The model under review builds one solid part; all positions refer to its coordinate system, in mm. Face numbers are marked on the shaded views. A direction names the side the tool comes from. Coordinates: 2 decimals unless noted, no trailing zeros. Loops run counter-clockwise (first coordinate to the right, second up) from the corner with the lowest first, then second, coordinate; pieces in that order, holes last. Notation, with made-up numbers: M -21.5,35.5 L 21.5,35.5 A27 cw 21.5,64.5 Z; hole C 82,36 d11. An arc over 180 degrees is marked long. Return JSON: item names as keys, results as strings.
```python
from build123d import *

# Parameters (mm, degrees)
F0_R     = 4
F1_DEPTH = 6
F3_SIZE  = 0.5
F4_R     = 1
F2_R     = 3
F5_DEPTH = 25
F6_SIZE  = 1.5


with BuildPart() as f1:
    # F0 (on Front) → F1 (new body)
    with BuildSketch(Plane.XZ):
        Polygon((0, 7.5055534995), (-6.5, 3.7527767497), (-6.5, -3.7527767497), (0, -7.5055534995), (6.5, -3.7527767497), (6.5, 3.7527767497), align=None)
        Circle(F0_R, mode=Mode.SUBTRACT)
        Circle(F0_R)
    extrude(amount=-F1_DEPTH)

    # F3
    f3_edges = [f1.edges().sort_by_distance(p)[0] for p in [
        (6.5, 0, 0),
        (-3.25, 0, 5.629165),
        (-6.5, 0, 0),
        (-3.25, 0, -5.629165),
        (3.25, 0, -5.629165),
        (-3.25, 6, 5.629165),
        (-6.5, 6, 0),
        (-3.25, 6, -5.629165),
        (3.25, 6, -5.629165),
        (6.5, 6, 0),
        (3.25, 6, 5.629165),
    ]]
    chamfer(f3_edges, length=F3_SIZE)

    # F4
    f4_edges = [f1.edges().sort_by_distance(p)[0] for p in [
        (0, 3, 7.505553),
        (-6.5, 3, 3.752777),
        (6.5, 3, 3.752777),
        (-6.5, 3, -3.752777),
        (0, 3, -7.505553),
        (6.5, 3, -3.752777),
    ]]
    fillet(f4_edges, radius=F4_R)

    # F2 (on face) → F5 (join)
    with BuildSketch(Plane.XZ):
        Circle(F2_R)
    extrude(amount=F5_DEPTH)

    # F6
    f6_edges = [f1.edges().sort_by_distance(p)[0] for p in [
        (-3, -25, 0),
    ]]
    chamfer(f6_edges, length=F6_SIZE)


solid = f1.part
```
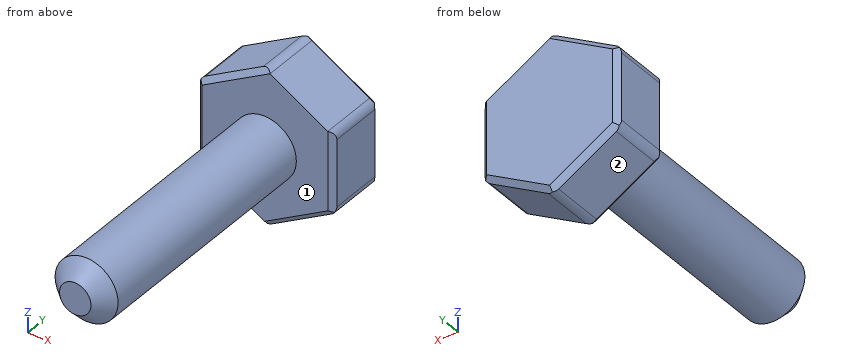
1. Add section B-B on x = -5. Give the boundary of the cut face in (y, z).
Check values:
{"outline": "M 0,-4.04 L 0.5,-4.62 L 5.5,-4.62 L 6,-4.04 L 6,4.04 L 5.5,4.62 L 0.5,4.62 L 0,4.04 Z"}
2. Add section A-A on z = 0. Give the boundary of the cut face in (x, y).
Check values:
{"outline": "M -6.5,0.5 L -6,0 L -3,0 L -3,-23.5 L -1.5,-25 L 1.5,-25 L 3,-23.5 L 3,0 L 6,0 L 6.5,0.5 L 6.5,5.5 L 6,6 L -6,6 L -6.5,5.5 Z"}
3. Add section D-D on z = -6. Give the boundary of the cut face in (x, y).
Check values:
{"outline": "M -2.61,0.5 L -1.61,0 L 1.61,0 L 2.61,0.5 L 2.61,5.5 L 1.61,6 L -1.61,6 L -2.61,5.5 Z"}
4. Machinability: for the marked faces 1 and 2, which of the approach directions +Z, -Z, +X, -X, +Y, -Y give a long, thin tool a straight path to every point of the face, cutting with its end or side? Answer none if there is none.
Check values:
{"face 1": "-Y", "face 2": "-Z, -X, +Y, -Y"}
5. Add section C-C on y = -23. Give the boundary of the cut face in (x, z), plus the area to 3 significant figures.
Check values:
{"outline": "C 0,0 d6", "area": "28.3 mm²"}
6. To check wall thickness, follow line 1 (Y direction, x = 0.25, z = 3.25); line 2 (Y direction, x = -1.75, z = -0.5); line 3 (X direction, y = -17, z = 0.5). State the ranges of each line that lie inside material, in increasing order.
Check values:
{"line 1": "0 to 6", "line 2": "-24.68 to 6", "line 3": "-2.96 to 2.96"}
7. Insertion check: pin 1 Ø3 at (y, z) = (-14.5, 2.5) entering from -X; pin 2 Ø1 at (y, z) = (-7.5, 1) entering from -X; pin 3 Ø2 at (x, z) = (-1, -4.5) entering from -Y. Each pin has a flat end and moves straight along its axis. Give the tip position at first contact, or say it passes through.
Check values:
{"pin 1": "x = -2.83", "pin 2": "x = -2.96", "pin 3": "y = 0"}
